Verification items for the finished model (mm, model axes). A direction names the side the tool comes from. Coordinates: 2 decimals unless noted, no trailing zeros. Order: outer loops, then holes, each group sorted by start corner. A loop starts at its lowest first (then second) coordinate and runs counter-clockwise, first axis right, second up. Notation, with made-up numbers: M 45,63.25 L 77,63.25 A24 cw 77,87.25 Z; hole C 0,86 d1. An arc over 180 degrees is marked long. Answer as a JSON object with one key per item and string values. Group by question number.
(1) Cross-section at C-C (z = 1.3). Enter the section's corners in (x, y), plus the area to 3 significant figures.
(2) Mould release check, pull along X, two halves, no side actions. Record for faces 1 (the face through (-13.6, -3, 2)), 2 (the face through (-0.2, -8.3, 5)), 3 (the face through (13.6, -3, 2)), 4 (the face through (12.23, -3.01, 2.05)): released by +X, released by -X, zero draft, split by the parting line, or undercut.
(3) Cross-section at B-B (y = -3). Enter the section's corners in (x, z).
(4) Material ranges on line 1 (X direction, y = -4.25, z = 2.5); line 2 (Z direction, x = 10.8, y = -1.25); line 3 (X direction, y = -3.75, z = 2.5), recorded low to high.
(5) Cross-section at D-D (y = -7.5). Enter the section's corners in (x, z), plus the area to 3 significant figures.
(6) Cross-section at A-A (x = -10.8). Enter the section's corners in (y, z), plus the area to 3 significant figures.
(7) Gauge pin test, flat ends, axial feed: pin 1 Ø1.8 at (x, z) = (-10.8, 2.5) entering from +Y; pin 2 Ø1.5 at (x, z) = (11.5, 3.5) entering from -Y. Record the tip position at first contact, or that the pin passes through.
(8) Access from +Z, -Z, +X, -X, +Y, -Y to the whole of each face (thin tool, end or side, straight path). Record for faces 5 (the face through (-10.8, -6.1, 0.8)), 6 (the face through (10.8, 0, 0.8)), 7 (the face through (10.8, -6.1, 0.8)).
from build123d import *

# Parameters (mm, degrees)
BOSS_EXTRUDE1_DEPTH = 5
SKETCH3_R           = 1.5
CUT_EXTRUDE1_DEPTH  = 10


with BuildPart() as part:
    # Sketch2 → Boss-Extrude1 (new body)
    with BuildSketch(Plane.XY):
        with BuildLine():
            ThreePointArc((-8, -6), (0, -10), (8, -6))
            Line((8, -6), (8, -6.1))
            Line((8, -6.1), (13.6, -6.1))
            Line((13.6, -6.1), (13.6, 0))
            Line((13.6, 0), (8, 0))
            ThreePointArc((8, 0), (0, -8), (-8, 0))
            Line((-8, 0), (-13.6, 0))
            Line((-13.6, 0), (-13.6, -6.1))
            Line((-13.6, -6.1), (-8, -6.1))
            Line((-8, -6.1), (-8, -6))
        make_face()
    extrude(amount=BOSS_EXTRUDE1_DEPTH)

    # Sketch3 → Cut-Extrude1 (cut)
    with BuildSketch(Plane(origin=(0, 0, 0), x_dir=(1, 0, 0), z_dir=(0, 1, 0))):
        with Locations((-10.8, -2.5)):
            Circle(SKETCH3_R)
        with Locations((10.8, -2.5)):
            Circle(SKETCH3_R)
    extrude(amount=-CUT_EXTRUDE1_DEPTH, mode=Mode.SUBTRACT)


solid = part.part
Taken from the geometry:
{
 "1": {"outline": "M -13.6,-6.1 L -11.7,-6.1 L -11.7,0 L -13.6,0 Z; M -9.9,-6.1 L -8,-6.1 L -8,-6 A10 ccw 8,-6 L 8,-6.1 L 9.9,-6.1 L 9.9,0 L 8,0 A8 cw -8,0 L -9.9,0 Z; M 11.7,-6.1 L 13.6,-6.1 L 13.6,0 L 11.7,0 Z", "area": "86.6 mm²"},
 "2": {"face 1": "released by -X", "face 2": "zero draft", "face 3": "released by +X", "face 4": "undercut"},
 "3": {"outline": "M -13.6,0 L -7.42,0 L -7.42,5 L -13.6,5 Z; M 7.42,0 L 13.6,0 L 13.6,5 L 7.42,5 Z; hole C -10.8,2.5 d3; hole C 10.8,2.5 d3"},
 "4": {"line 1": "x = -13.6 to -12.3, -9.3 to -6.78, 6.78 to 9.3, 12.3 to 13.6", "line 2": "z = 0 to 1, 4 to 5", "line 3": "x = -13.6 to -12.3, -9.3 to -7.07, 7.07 to 9.3, 12.3 to 13.6"},
 "5": {"outline": "M -6.61,0 L -2.78,0 L -2.78,5 L -6.61,5 Z; M 2.78,0 L 6.61,0 L 6.61,5 L 2.78,5 Z", "area": "38.3 mm²"},
 "6": {"outline": "M -6.1,0 L 0,0 L 0,1 L -6.1,1 Z; M -6.1,4 L 0,4 L 0,5 L -6.1,5 Z", "area": "12.2 mm²"},
 "7": {"pin 1": "passes through", "pin 2": "stops at y = -6.1"},
 "8": {"face 5": "+Z, -Z, -X, -Y", "face 6": "+Z, -Z, +X, -X, +Y", "face 7": "+Z, -Z, +X, -Y"}
}
